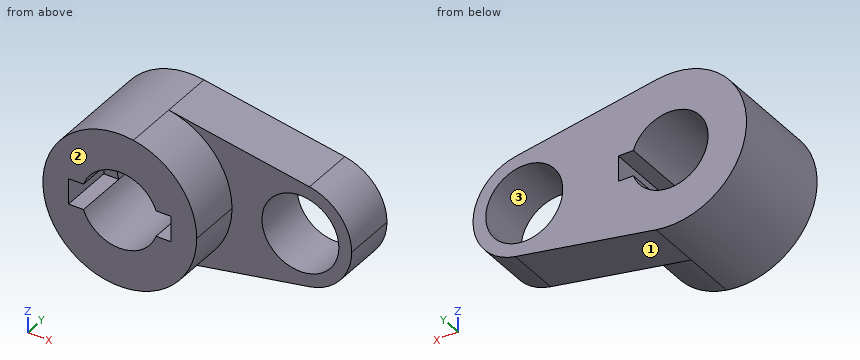
```python
from build123d import *

# Parameters (mm, degrees)
F0_R     = 14.2875
F1_DEPTH = 20
F2_DEPTH = 40


with BuildPart() as f1:
    # F0 (on Front) → F1 (new body)
    with BuildSketch(Plane.XZ):
        with BuildLine():
            ThreePointArc((5.042647, 28.126541), (21.916025, 18.336262), (28.575, 0))
            ThreePointArc((28.575, 0), (21.916025, -18.336262), (5.042647, -28.126541))
            Line((5.042647, -28.126541), (57.336765, -18.751028))
            ThreePointArc((57.336765, -18.751028), (34.925, 0), (57.336765, 18.751028))
            Line((57.336765, 18.751028), (5.042647, 28.126541))
        make_face()
        with BuildLine():
            ThreePointArc((73.025, 0), (68.585683, 12.224174), (57.336765, 18.751028))
            ThreePointArc((57.336765, 18.751028), (34.925, 0), (57.336765, -18.751028))
            ThreePointArc((57.336765, -18.751028), (68.585683, -12.224174), (73.025, 0))
        make_face()
        with Locations((53.975, 0)):
            Circle(F0_R, mode=Mode.SUBTRACT)
        with BuildLine():
            ThreePointArc((5.042647, -28.126541), (21.916025, -18.336262), (28.575, 0))
            ThreePointArc((28.575, 0), (21.916025, 18.336262), (5.042647, 28.126541))
            ThreePointArc((5.042647, 28.126541), (-28.575, 0), (5.042647, -28.126541))
        make_face()
        with BuildLine():
            ThreePointArc((-13.470384, 4.7625), (0, 14.2875), (13.470384, 4.7625))
            Line((13.470384, 4.7625), (19.05, 4.7625))
            Line((19.05, 4.7625), (19.05, -4.7625))
            Line((19.05, -4.7625), (13.470384, -4.7625))
            ThreePointArc((13.470384, -4.7625), (0, -14.2875), (-13.470384, -4.7625))
            Line((-13.470384, -4.7625), (-19.05, -4.7625))
            Line((-19.05, -4.7625), (-19.05, 4.7625))
            Line((-19.05, 4.7625), (-13.470384, 4.7625))
        make_face(mode=Mode.SUBTRACT)
        with BuildLine():
            ThreePointArc((-13.470384, -4.7625), (-14.2875, 0), (-13.470384, 4.7625))
            Line((-13.470384, 4.7625), (-19.05, 4.7625))
            Line((-19.05, 4.7625), (-19.05, -4.7625))
            Line((-19.05, -4.7625), (-13.470384, -4.7625))
        make_face()
    extrude(amount=F1_DEPTH)

    # F0 (on Front) → F2 (join)
    with BuildSketch(Plane.XZ):
        with BuildLine():
            ThreePointArc((5.042647, -28.126541), (21.916025, -18.336262), (28.575, 0))
            ThreePointArc((28.575, 0), (21.916025, 18.336262), (5.042647, 28.126541))
            ThreePointArc((5.042647, 28.126541), (-28.575, 0), (5.042647, -28.126541))
        make_face()
        with BuildLine():
            ThreePointArc((-13.470384, 4.7625), (0, 14.2875), (13.470384, 4.7625))
            Line((13.470384, 4.7625), (19.05, 4.7625))
            Line((19.05, 4.7625), (19.05, -4.7625))
            Line((19.05, -4.7625), (13.470384, -4.7625))
            ThreePointArc((13.470384, -4.7625), (0, -14.2875), (-13.470384, -4.7625))
            Line((-13.470384, -4.7625), (-19.05, -4.7625))
            Line((-19.05, -4.7625), (-19.05, 4.7625))
            Line((-19.05, 4.7625), (-13.470384, 4.7625))
        make_face(mode=Mode.SUBTRACT)
    extrude(amount=F2_DEPTH)


solid = f1.part
```
Geometry check sheet. Reference: the model listing, model coordinates, mm. Face numbers are marked on the shaded views. Coordinates: 2 decimals unless noted, no trailing zeros. Write each loop counter-clockwise with the first axis right and the second up, starting at its lowest first coordinate (ties: lowest second). Pieces come first, ordered by that corner, then holes. Notation, with made-up numbers: M 3,82.25 L 7,82.25 A30 ccw 7,114.25 Z; hole C -27,-2.5 d9. An arc over 180 degrees is marked long. Use one line per item in the form item = value. Start each with the question number.
1) Section check D-D on x = 66.5. Enter the section's corners in (y, z), and give its area (3 significant figures).
2) Section check A-A on y = -2.5. State how many separate pieces and enclosed holes the cut face has, and give its area (3 significant figures).
3) Section check B-B on x = 0. Enter the section's corners in (y, z) (1 decimal).
4) Thickness scan on probe 1 along Z at (x, y) = (16, -38); probe 2 along Z at (x, y) = (-3.5, -23.5); probe 3 along X at (y, z) = (-29, -4.5). Record the ranges inside material, lowest first. Write a range as from..to.
5) Go/stop test with flat-tipped pins: pin 1 Ø12 at (x, y) = (-11, -29) entering from -Z; pin 2 Ø4 at (y, z) = (-31, 12) entering from -X; pin 3 Ø1.7 at (x, y) = (16.5, -25) entering from +Z; pin 4 Ø23 at (x, z) = (53.975, 0) entering from -Y. Record where each tip stops, or that it passes through.
6) Release check for a two-part mould opening along X. For the marked faces 1, 2 and 3 record: pulls with the +X half, pulls with the -X half, needs draft (parallel to the pull), parting line crosses it, or undercut.
Responses:
q1.outline = M -20,-14.35 L 0,-14.35 L 0,-6.87 L -20,-6.87 Z; M -20,6.87 L 0,6.87 L 0,14.35 L -20,14.35 Z
q1.area = 299 mm2
q2.separate_pieces = 1
q2.enclosed_holes = 2
q2.area = 3,130 mm2
q3.outline = M -40,-28.6 L 0,-28.6 L 0,-14.3 L -40,-14.3 Z; M -40,14.3 L 0,14.3 L 0,28.6 L -40,28.6 Z
q4.probe_1 = -23.68..-4.76, 4.76..23.68
q4.probe_2 = -28.36..-13.85, 13.85..28.36
q4.probe_3 = -28.22..-19.05, 19.05..28.22
q5.pin_1 = -28.13
q5.pin_2 = -26.77
q5.pin_3 = 23.91
q5.pin_4 = through
q6.face_1 = pulls with the +X half
q6.face_2 = needs draft
q6.face_3 = undercut
